Source: CAD feature listing. Evaluate the final solid. Frame: model axes, mm. Give positions to 0.01 mm unless a question says otherwise; leave off trailing zeros. Loops run counter-clockwise (first coordinate to the right, second up) from the corner with the lowest first, then second, coordinate; pieces in that order, holes last. Notation, with made-up numbers: (-4.5, -29) -> (25.5, -29) arc R23 cw to (25.5, -20) -> close; hole circle Ø7 at (70, -31). An arc over 180 degrees is marked (long way). Put each result on its own line as item: value.
```python
from build123d import *

# Parameters (mm, degrees)
SKETCH2_R          = 1.75
CUT_EXTRUDE1_DEPTH = 10


with BuildPart() as part:
    # Sketch1 → Revolve1 (revolve)
    with BuildSketch(Plane.XY, mode=Mode.PRIVATE) as revolve1_sk:
        Polygon((-18, 30), (-18, -26.5), (-25, -26.5), (-25, -30), (-16, -30), (-16, 30), align=None)
    revolve(revolve1_sk.sketch.rotate(Axis((0, 40.25, 0), (0, -1, 0)), 270), axis=Axis((0, 40.25, 0), (0, -1, 0)))

    # Sketch2 → Cut-Extrude1 (cut)
    with BuildSketch(Plane(origin=(0, -26.5, 0), x_dir=(1, 0, 0), z_dir=(0, 1, 0))):
        with Locations(Location((0, 21.25, 0), (0, 0, 270))):
            Circle(SKETCH2_R)
        with Locations(Location((15.0260191, 15.0260191, 0), (0, 0, 270))):
            Circle(SKETCH2_R)
        with Locations(Location((21.25, 0, 0), (0, 0, 270))):
            Circle(SKETCH2_R)
        with Locations(Location((15.0260191, -15.0260191, 0), (0, 0, 270))):
            Circle(SKETCH2_R)
        with Locations(Location((0, -21.25, 0), (0, 0, 270))):
            Circle(SKETCH2_R)
        with Locations(Location((-15.0260191, -15.0260191, 0), (0, 0, 270))):
            Circle(SKETCH2_R)
        with Locations(Location((-21.25, 0, 0), (0, 0, 270))):
            Circle(SKETCH2_R)
        with Locations(Location((-15.0260191, 15.0260191, 0), (0, 0, 270))):
            Circle(SKETCH2_R)
    extrude(amount=-CUT_EXTRUDE1_DEPTH, mode=Mode.SUBTRACT)


solid = part.part
```
(1) Section C-C on z = -7. Return loops of the section in (x, y), then the cut area to 3 significant figures.
Calculated:
outline: (-24, -30) -> (-14.39, -30) -> (-14.39, 30) -> (-16.58, 30) -> (-16.58, -26.5) -> (-24, -26.5) -> close; (14.39, -30) -> (24, -30) -> (24, -26.5) -> (16.58, -26.5) -> (16.58, 30) -> (14.39, 30) -> close
area: 315 mm²
(2) First-contact query: P1, Ø4, axis at x = 0, z = 21.25, coming from the +Y side; P2, Ø2, axis at x = 0, z = -21.25, coming from the -Y side; P3, Ø4, axis at y = -7, z = -4.5, coming from the -X side; P4, Ø4, axis at x = -21.25, z = 0, coming from the -Y side. Flat tips, straight axial feed; report the tip coordinate or a pass-through.
Calculated:
P1: stops at y = -26.5
P2: passes through
P3: stops at x = -17.83
P4: stops at y = -30
(3) Draft query along Z for faces 1 (the cylindrical face through (-5.407, 1.354, 17.169)), 2 (the cylindrical face through (-16.58, -28.23, -14.22)), 3 (the flat face through (17, -26.5, 8)). Return one class per face: released by +Z, released by -Z, zero draft, split by the parting line, or undercut.
Calculated:
face 1: split by the parting line
face 2: undercut
face 3: zero draft
(4) Line query: probe 1 along Z at (x, y) = (-9, -10.5); probe 2 along Y at (x, z) = (17, -7.5); probe 3 along Z at (x, y) = (7.5, -27.5). Output: solid intervals per line, ascending. Write a range as from..to.
Calculated:
probe 1: z = -15.59..-13.23, 13.23..15.59
probe 2: y = -30..-26.5
probe 3: z = -23.85..-14.13, 14.13..23.85
(5) Section A-A on x = 0. Return loops of the section in (y, z), then the cut area to 4 significant figures.
Calculated:
outline: (-30, -25) -> (-26.5, -25) -> (-26.5, -23) -> (-30, -23) -> close; (-30, -19.5) -> (-26.5, -19.5) -> (-26.5, -18) -> (30, -18) -> (30, -16) -> (-30, -16) -> close; (-30, 16) -> (30, 16) -> (30, 18) -> (-26.5, 18) -> (-26.5, 19.5) -> (-30, 19.5) -> close; (-30, 23) -> (-26.5, 23) -> (-26.5, 25) -> (-30, 25) -> close
area: 264.5 mm²
(6) Section B-B on z = 0. Return loops of the section in (x, y), then the cut area to 4 significant figures.
Calculated:
outline: (-25, -30) -> (-23, -30) -> (-23, -26.5) -> (-25, -26.5) -> close; (-19.5, -30) -> (-16, -30) -> (-16, 30) -> (-18, 30) -> (-18, -26.5) -> (-19.5, -26.5) -> close; (16, -30) -> (19.5, -30) -> (19.5, -26.5) -> (18, -26.5) -> (18, 30) -> (16, 30) -> close; (23, -30) -> (25, -30) -> (25, -26.5) -> (23, -26.5) -> close
area: 264.5 mm²
(7) Section D-D on x = -5. Return loops of the section in (y, z), then the cut area to 3 significant figures.
Calculated:
outline: (-30, -24.49) -> (-26.5, -24.49) -> (-26.5, -17.29) -> (30, -17.29) -> (30, -15.2) -> (-30, -15.2) -> close; (-30, 15.2) -> (30, 15.2) -> (30, 17.29) -> (-26.5, 17.29) -> (-26.5, 24.49) -> (-30, 24.49) -> close
area: 302 mm²
